```python
from build123d import *

# Parameters (mm, degrees)
BOSS_EXTRUDE1_DEPTH = 59.69
SKETCH2_W           = 1.5875
SKETCH2_H           = 6.35
BOSS_EXTRUDE2_DEPTH = 1.5875


with BuildPart() as part:
    # Sketch1 → Boss-Extrude1 (new body)
    with BuildSketch(Plane(origin=(0, 0, 0), x_dir=(0, 0, -1), z_dir=(1, 0, 0))):
        with BuildLine():
            Line((0.590873303, -4.466173809), (0.136355378, -10.799886264))
            Line((0.136355378, -10.799886264), (0, -12.7))
            Line((0, -12.7), (1.619880116, -12.30567041))
            Line((1.619880116, -12.30567041), (2.174301417, -4.579803291))
            Line((2.174301417, -4.579803291), (2.409882648, -1.296976159))
            ThreePointArc((2.409882648, -1.296976159), (1.441524141, 1.753522136), (1.266539623, 4.949244036))
            Line((1.266539623, 4.949244036), (0.590873303, -4.466173809))
        make_face()
    extrude(amount=BOSS_EXTRUDE1_DEPTH)

    # Sketch2 → Boss-Extrude2 (add)
    with BuildSketch(Plane(origin=(0, -0.065066628, -0.906704203), x_dir=(1, 0, 0), z_dir=(0, 0.07157762605528778, 0.9974350321942224))):
        with Locations((-0.79375, -7.587424909)):
            Rectangle(SKETCH2_W, SKETCH2_H)
        with Locations((60.48375, -7.587424909)):
            Rectangle(SKETCH2_W, SKETCH2_H)
    extrude(amount=-BOSS_EXTRUDE2_DEPTH)


solid = part.part
```
Geometry check sheet. Reference: the model listing, model coordinates, mm. A direction names the side the tool comes from. Give positions to 0.01 mm unless a question says otherwise; leave off trailing zeros. Write each loop counter-clockwise with the first axis right and the second up, starting at its lowest first coordinate (ties: lowest second). Pieces come first, ordered by that corner, then holes.
1) Section check C-C, the plane y = 2.75. Record the boundary of the cut face in (x, z), and give its area (3 significant figures).
2) Section check B-B, the plane y = -9.75. Record the boundary of the cut face in (x, z), and give its area (3 significant figures).
3) Section check A-A, the plane x = 19.5. Record the boundary of the cut face in (y, z), and give its area (3 significant figures).
4) Section check D-D, the plane y = -0.5. Record the boundary of the cut face in (x, z).
5) Access from +Z, -Z, +X, -X, +Y, -Y to the whole of each face (thin tool, end or side, straight path). Record for faces 1 (the flat face through (60.473, -4.522, -1.372)), 2 (the flat face through (-0.805, -10.856, -0.917)), 3 (the flat face through (-0.805, -4.522, -1.372)), 4 (the flat face through (60.473, -10.856, -0.917)).
6) Material ranges on L1, parallel to X at y = -1, z = -1.35; L2, parallel to Z at x = 19, y = -10; L3, parallel to Z at x = 40, y = -1, recorded low to high.
7) Gauge pin test, flat ends, axial feed: pin 1 (0.5 mm diameter, centred on y = -11.5, z = -1, fed in from -X); pin 2 (0.9 mm diameter, centred on y = -1.5, z = -1.5, fed in from +X). Record the tip position at first contact, or that the pin passes through.
Computed:
1. outline: (0, -1.3) - (59.69, -1.3) - (59.69, -1.11) - (0, -1.11) - close
1. area: 11.4 mm2
2. outline: (-1.59, -1.8) - (61.28, -1.8) - (61.28, -0.21) - (-1.59, -0.21) - close
2. area: 100 mm2
3. outline: (-12.7, 0) - (-12.31, -1.62) - (-1.3, -2.41) arc R12.7 cw to (4.95, -1.27) - close
3. area: 21.1 mm2
4. outline: (0, -2.07) - (59.69, -2.07) - (59.69, -0.88) - (0, -0.88) - close
5. face 1: -Z, +X, +Y
5. face 2: +Z, -X, -Y
5. face 3: -Z, -X, +Y
5. face 4: +Z, +X, -Y
6. L1: x = 0 to 59.69
6. L2: z = -1.79 to -0.19
6. L3: z = -2.28 to -0.84
7. pin 1: stops at x = 0
7. pin 2: stops at x = 59.69
